```python
from build123d import *

# Parameters (mm, degrees)
F0_W     = 61.8086736649
F0_H     = 40.3841938823
F1_DEPTH = 42.164
F2_T     = -5.08
F3_SIZE  = 5.07999
F4_SIZE  = 5.07999
F5_SIZE  = 5.07999


# Not quite as in the source:
# - a fillet or chamfer is up to 0.001 mm smaller than in the source, because OpenCascade refuses the exact size


with BuildPart() as f1:
    # F0 (on Top) → F1 (new body)
    with BuildSketch(Plane.XY):
        with Locations((-2.8439583257, 1.9907699898)):
            Rectangle(F0_W, F0_H)
    extrude(amount=F1_DEPTH)

    # F2
    f2_openings = [f1.faces().sort_by_distance(p)[0] for p in [
        (-2.843958, -18.201327, 21.082),
    ]]
    offset(amount=F2_T, openings=f2_openings)

    # F3 (size 5.08 in the source; OpenCascade refuses exactly that, so slightly less here)
    f3_edges = [f1.edges().sort_by_distance(p)[0] for p in [
        (-2.843958, -18.201327, 42.164),
    ]]
    chamfer(f3_edges, length=F3_SIZE)

    # F4 (size 5.08 in the source; OpenCascade refuses exactly that, so slightly less here)
    f4_edges = [f1.edges().sort_by_distance(p)[0] for p in [
        (-33.748295, -18.201327, 18.542005),
        (28.060379, -18.201327, 18.542005),
    ]]
    chamfer(f4_edges, length=F4_SIZE)

    # F5 (size 5.08 in the source; OpenCascade refuses exactly that, so slightly less here)
    f5_edges = [f1.edges().sort_by_distance(p)[0] for p in [
        (-2.843958, -18.201327, 0),
    ]]
    chamfer(f5_edges, length=F5_SIZE)


solid = f1.part
```
CAD build for the part. Positions are in the model's coordinates, mm. A direction names the side the tool comes from. Give positions to 0.01 mm unless a question says otherwise; leave off trailing zeros. Write each loop counter-clockwise with the first axis right and the second up, starting at its lowest first coordinate (ties: lowest second). Pieces come first, ordered by that corner, then holes. Notation, with made-up numbers: M 17.25,52.5 L 40.25,52.5 A16 cw 40.25,67.5 Z; hole C 88,55.25 d4. An arc over 180 degrees is marked long. Return JSON: item names as keys, results as strings. Group by question number.
(1) Band-saw the part on D-D (y = -14). Give the cut face in (x, z).
(2) Band-saw the part on A-A (y = -9.5). Give the cut face in (x, z).
(3) Flat gauge pin, fed straight in: pin 1 Ø16 at (x, z) = (-14.5, 21) entering from -Y. Where does the tip first touch, or does it go through?
(4) 3-axis set-ups, long thin cutter, end or side, ignore diameter. For faces 1 (the face through (-3.28, -15.7, 2.58)), 2 (the face through (-3, 0, 37.084)): which of +Z, -Z, +X, -X, +Y, -Y reach the whole face in a straight line?
(5) Mould opens along Z. For faces 3 (the face through (28.06, 4, 21)), 4 (the face through (-3, 0, 5.08)), 5 (the face through (-3, 5, 42.164)) say: pulls with the +Z half, pulls with the -Z half, needs draft (parallel to the pull), parting line crosses it, or undercut.
(6) Drill centre lines: L1, parallel to Z at x = -15.5, y = -6; L2, parallel to X at y = 7, z = 15; L3, parallel to Y at x = -10.5, z = 14.5. Where is each one in solid material? Low to high. Write a range as [from, to].
Entries:
{
 "1": {"outline": "M -32.87,0.88 L 27.18,0.88 L 27.18,41.29 L -32.87,41.29 Z; hole M -28.67,5.08 L 22.98,5.08 L 22.98,37.08 L -28.67,37.08 Z"},
 "2": {"outline": "M -33.75,0 L 28.06,0 L 28.06,42.16 L -33.75,42.16 Z; hole M -28.67,5.08 L 22.98,5.08 L 22.98,37.08 L -28.67,37.08 Z"},
 "3": {"pin 1": "stops at y = 17.1"},
 "4": {"face 1": "-Z, +X, -X, -Y", "face 2": "-Y"},
 "5": {"face 3": "needs draft", "face 4": "undercut", "face 5": "pulls with the +Z half"},
 "6": {"L1": "z = [0, 5.08], [37.08, 42.16]", "L2": "x = [-33.75, -28.67], [22.98, 28.06]", "L3": "y = [17.1, 22.18]"}
}
